Model file for the job. Use its own axes, mm. Face numbers are marked on the shaded views. Give positions to 0.01 mm unless a question says otherwise; leave off trailing zeros. Order: outer loops, then holes, each group sorted by start corner. A loop starts at its lowest first (then second) coordinate and runs counter-clockwise, first axis right, second up. Notation, with made-up numbers: M 42,41 L 49,41 A12 ccw 49,47 Z; hole C -20.5,61 d6. An arc over 180 degrees is marked long. Return JSON: item names as keys, results as strings. Group by question number.
1. Pin check, flat tips, straight feed: pin 1 (12 mm diameter, centred on x = -21, z = -14, fed in from -Y); pin 2 (15.5 mm diameter, centred on x = 0, z = 0, fed in from +Y). Stop position of each tip, or through.
2. Slice it at A-A on z = 0. List the corners of the cut face in (x, y).
3. Two-plate mould, pull along Z, no slides. Class the marked faces 1, 2 and 3: released by +Z, released by -Z, zero draft, split by the parting line, or undercut.
4. Wall check: probe 1 along X at (y, z) = (3.25, 0); probe 2 along X at (y, z) = (5.75, 3); probe 3 along Z at (x, y) = (4, 5). Give the ranges that are in metal, low to high. Write a range as [from, to].
5. Slice it at C-C on x = 0. List the corners of the cut face in (y, z), then the cut area to 4 significant figures.
6. Slice it at B-B on y = 2.25. List the corners of the cut face in (x, z), then the cut area to 3 significant figures.
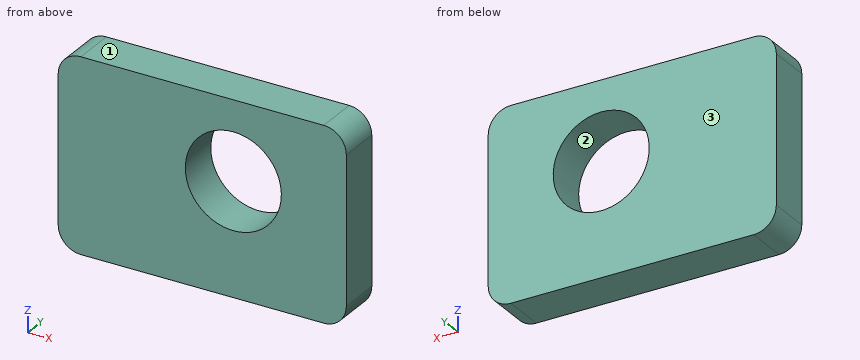
from build123d import *

# Parameters (mm, degrees)
SKETCH1_R           = 8.5
BOSS_EXTRUDE1_DEPTH = 7.5
FILLET1_R           = 4


with BuildPart() as part:
    # Sketch1 → Boss-Extrude1 (new body)
    with BuildSketch(Plane(origin=(0, 0, 0), x_dir=(1, 0, 0), z_dir=(0, 1, 0))):
        Polygon((-31, 0), (-31, 20), (20, 20), (20, 0), (20, -14), (-31, -14), align=None)
        with Locations(Location((0, 0, 0), (0, 0, 270))):
            Circle(SKETCH1_R, mode=Mode.SUBTRACT)
    extrude(amount=BOSS_EXTRUDE1_DEPTH)

    # Fillet1
    fillet1_edges = [part.edges().sort_by_distance(p)[0] for p in [
        (20, 3.75, 14),
        (-31, 3.75, 14),
        (-31, 3.75, -20),
        (20, 3.75, -20),
    ]]
    fillet(fillet1_edges, radius=FILLET1_R)


solid = part.part
Result:
{
 "1": {"pin 1": "stops at y = 0", "pin 2": "passes through"},
 "2": {"outline": "M -31,0 L -8.5,0 L -8.5,7.5 L -31,7.5 Z; M 8.5,0 L 20,0 L 20,7.5 L 8.5,7.5 Z"},
 "3": {"face 1": "released by +Z", "face 2": "undercut", "face 3": "zero draft"},
 "4": {"probe 1": "x = [-31, -8.5], [8.5, 20]", "probe 2": "x = [-31, -7.95], [7.95, 20]", "probe 3": "z = [-20, -7.5], [7.5, 14]"},
 "5": {"outline": "M 0,-20 L 7.5,-20 L 7.5,-8.5 L 0,-8.5 Z; M 0,8.5 L 7.5,8.5 L 7.5,14 L 0,14 Z", "area": "127.5 mm2"},
 "6": {"outline": "M -31,-16 A4 ccw -27,-20 L 16,-20 A4 ccw 20,-16 L 20,10 A4 ccw 16,14 L -27,14 A4 ccw -31,10 Z; hole C 0,0 d17", "area": "1,490 mm2"}
}
